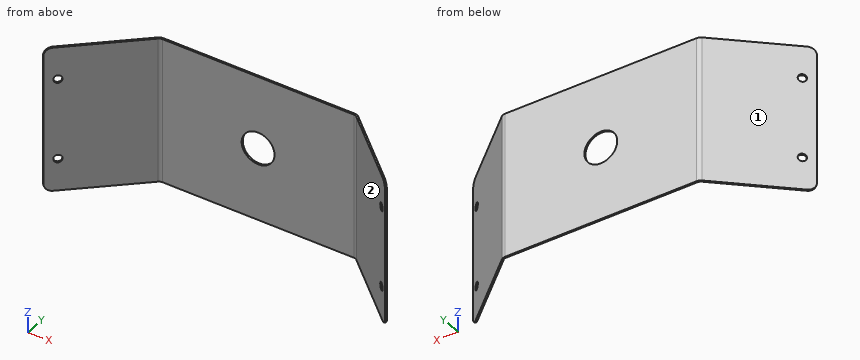
from build123d import *

# Parameters (mm, degrees)
ESBO_O1_W                 = 116.5
ESBO_O1_H                 = 90
FLANGE_BASE1_DEPTH        = 1
ARESTA_FLANGE1_DEPTH      = 90
ARESTA_FLANGE1_BEND_DEPTH = 90
CORTE_EXTRUS_O1_REACH     = 157.954
ESBO_O12_R                = 2.4
FILETE1_R                 = 5
CORTE_EXTRUS_O2_REACH     = 123.127
ESBO_O13_R                = 10


# Sheet-metal steps are written as plain solids
with BuildPart() as part:
    # Esbo_o1 → Flange-base1 (new body)
    with BuildSketch(Plane(origin=(0, 0, 0), x_dir=(1, 0, 0), z_dir=(0, 1, 0))):
        Rectangle(ESBO_O1_W, ESBO_O1_H)
    extrude(amount=-FLANGE_BASE1_DEPTH)

    # Aresta-Flange1 section (across the edge) → Aresta-Flange1 (add)
    with BuildSketch(Plane(origin=(59.401592105, -1, -45), x_dir=(-0.6691306063588541, -0.7431448254773979, 0), z_dir=(0, 0, 1))):
        with BuildLine():
            Line((-1, 1.151592105), (-1, 60))
            Line((-1, 60), (0, 60))
            Line((0, 60), (0, 1.151592105))
            ThreePointArc((0, 1.151592105), (0.199258721, 0.076488256), (0.770565524, -0.855799714))
            Line((0.770565524, -0.855799714), (0.027420698, -1.52493032))
            ThreePointArc((0.027420698, -1.52493032), (-0.734321706, -0.281879693), (-1, 1.151592105))
        make_face()
    extrude(amount=ARESTA_FLANGE1_DEPTH)

    # Aresta-Flange1 section 2 (across the edge) → Aresta-Flange1 bend (add)
    with BuildSketch(Plane(origin=(-59.401592105, -1, 45), x_dir=(0.6691306063588541, -0.7431448254773979, 0), z_dir=(0, 0, -1))):
        with BuildLine():
            Line((-1, 1.151592105), (-1, 60))
            Line((-1, 60), (0, 60))
            Line((0, 60), (0, 1.151592105))
            ThreePointArc((0, 1.151592105), (0.199258721, 0.076488256), (0.770565524, -0.855799714))
            Line((0.770565524, -0.855799714), (0.027420698, -1.52493032))
            ThreePointArc((0.027420698, -1.52493032), (-0.734321706, -0.281879693), (-1, 1.151592105))
        make_face()
    extrude(amount=ARESTA_FLANGE1_BEND_DEPTH)

    # Esbo_o12 → Corte-extrus_o1 (cut, up to next)
    with BuildSketch(Plane(origin=(26.768087142, 29.728972578, 0), x_dir=(0.7431448254773978, -0.6691306063588544, 0), z_dir=(0.6691306063588544, 0.7431448254773978, 0)), mode=Mode.PRIVATE) as corte_extrus_o1_sk1:
        with Locations(Location((97.313116404, -25, 0), (0, 0, 180))):
            Circle(ESBO_O12_R)
    corte_extrus_o1_tool1 = extrude(corte_extrus_o1_sk1.sketch, amount=-CORTE_EXTRUS_O1_REACH, mode=Mode.PRIVATE) & part.part
    # Esbo_o12 → Corte-extrus_o1 (cut, up to next)
    with BuildSketch(Plane(origin=(26.768087142, 29.728972578, 0), x_dir=(0.7431448254773978, -0.6691306063588544, 0), z_dir=(0.6691306063588544, 0.7431448254773978, 0)), mode=Mode.PRIVATE) as corte_extrus_o1_sk2:
        with Locations(Location((97.313116404, 25, 0), (0, 0, 180))):
            Circle(ESBO_O12_R)
    corte_extrus_o1_tool2 = extrude(corte_extrus_o1_sk2.sketch, amount=-CORTE_EXTRUS_O1_REACH, mode=Mode.PRIVATE) & part.part
    corte_extrus_o1_1 = corte_extrus_o1_tool1.solids().sort_by_distance((99.085826, -35.386212, 25))[0]
    add(corte_extrus_o1_1, mode=Mode.SUBTRACT)
    corte_extrus_o1_2 = corte_extrus_o1_tool2.solids().sort_by_distance((99.085826, -35.386212, -25))[0]
    add(corte_extrus_o1_2, mode=Mode.SUBTRACT)
    corte_extrus_o1 = corte_extrus_o1_1 + corte_extrus_o1_2  # Corte-extrus_o1 as one shape, for the pattern or mirror that repeats it

    # Espelhar1: Corte-extrus_o1 across plane
    add(corte_extrus_o1.mirror(Plane(origin=(0, 0, 0), x_dir=(0, 0, 1), z_dir=(1, 0, 0))), mode=Mode.SUBTRACT)

    # Filete1
    filete1_edges = [part.edges().sort_by_distance(p)[0] for p in [
        (104.324846937, -40.776263969, -45),
        (104.324846937, -40.776263969, 45),
        (-104.324846937, -40.776263969, 45),
        (-104.324846937, -40.776263969, -45),
    ]]
    fillet(filete1_edges, radius=FILETE1_R)

    # Esbo_o13 → Corte-extrus_o2 (cut, up to next)
    with BuildSketch(Plane(origin=(0, 0, 0), x_dir=(1, 0, 0), z_dir=(0, 1, 0)), mode=Mode.PRIVATE) as corte_extrus_o2_sk1:
        with Locations(Location((0, 0, 0), (0, 0, 270))):
            Circle(ESBO_O13_R)
    corte_extrus_o2_tool1 = extrude(corte_extrus_o2_sk1.sketch, amount=-CORTE_EXTRUS_O2_REACH, mode=Mode.PRIVATE) & part.part
    add(corte_extrus_o2_tool1.solids().sort_by_distance((0, 0, 0))[0], mode=Mode.SUBTRACT)


solid = part.part
Model file for the job. Use its own axes, mm. Face numbers are marked on the shaded views. A direction names the side the tool comes from. Round coordinates to 2 decimals unless told otherwise and drop trailing zeros. Order: outer loops, then holes, each group sorted by start corner. A loop starts at its lowest first (then second) coordinate and runs counter-clockwise, first axis right, second up.
(1) Drill centre lines: line 1 (X direction, y = -0.55, z = 0); line 2 (X direction, y = -10.5, z = -1.5); line 3 (Y direction, x = 22, z = -31.5). Where is each one in solid material? Low to high.
(2) Band-saw the part on B-B (x = 0). List the corners of the cut face in (y, z), then the cut area to 3 significant figures.
(3) Band-saw the part on A-A (z = 8). List the corners of the cut face in (x, y).
(4) Pin check, flat tips, straight feed: pin 1 (5 mm diameter, centred on x = 83, z = 2, fed in from -Y); pin 2 (1 mm diameter, centred on x = 69.5, z = -9.5, fed in from -Y); pin 3 (3 mm diameter, centred on y = -19.5, z = 14.5, fed in from -X). Stop position of each tip, or through.
(5) Band-saw the part on D-D (x = -64). List the corners of the cut face in (y, z), then the cut area to 3 significant figures.
(6) 3-axis set-ups, long thin cutter, end or side, ignore diameter. For the marked faces 1 and 2: which of +Z, -Z, +X, -X, +Y, -Y reach the whole face in a straight line?
(7) Band-saw the part on C-C (y = -27). List the corners of the cut face in (x, z).
Verdict:
1. line 1: x = -60.27 to -10, 10 to 60.27
1. line 2: x = -71.45 to -69.95, 69.95 to 71.45
1. line 3: y = -1 to 0
2. outline: (-1, -45) - (0, -45) - (0, -10) - (-1, -10) - close; (-1, 10) - (0, 10) - (0, 45) - (-1, 45) - close
2. area: 70.0 mm2
3. outline: (-104.66, -40.4) - (-103.99, -41.15) - (-60.26, -1.77) arc R3 cw to (-58.25, -1) - (-6, -1) - (-6, 0) - (-58.25, 0) arc R4 ccw to (-60.93, -1.03) - close; (6, -1) - (58.25, -1) arc R3 cw to (60.26, -1.77) - (103.99, -41.15) - (104.66, -40.4) - (60.93, -1.03) arc R4 ccw to (58.25, 0) - (6, 0) - close
4. pin 1: stops at y = -24.5
4. pin 2: stops at y = -10.54
4. pin 3: stops at x = -83.11
5. outline: (-5.14, -45) - (-3.79, -45) - (-3.79, 45) - (-5.14, 45) - close
5. area: 121 mm2
6. face 1: +Z, -Z, -X, +Y
6. face 2: +Z, -Z, -Y
7. outline: (-89.77, -45) - (-88.28, -45) - (-88.28, 45) - (-89.77, 45) - close; (88.28, -45) - (89.77, -45) - (89.77, 45) - (88.28, 45) - close
